Geometry check sheet. Reference: the model listing, model coordinates, mm. A direction names the side the tool comes from. Round coordinates to 2 decimals unless told otherwise and drop trailing zeros. Loops run counter-clockwise (first coordinate to the right, second up) from the corner with the lowest first, then second, coordinate; pieces in that order, holes last. Notation, with made-up numbers: (30.5, 70) - (73.5, 70) arc R26 ccw to (73.5, 105) - close; hole circle Ø6 at (48, -37). An arc over 180 degrees is marked (long way). Answer in a Markdown table with one row per item. Add a question column.
```python
from build123d import *

# Parameters (mm, degrees)
SKETCH4_W           = 17.9705
SKETCH4_H           = 57.023
SKETCH4_W_2         = 1.5875
SKETCH4_H_2         = 16.51
BOSS_EXTRUDE3_DEPTH = 9.906
SKETCH6_W           = 0.762
SKETCH6_H           = 36.957
REVOLVE2_ANGLE      = 345
SKETCH8_W           = 0.635
SKETCH8_H           = 4.826
BOSS_EXTRUDE4_DEPTH = 6.985


with BuildPart() as part:
    # Sketch4 → Revolve1 (revolve)
    with BuildSketch(Plane(origin=(0, 0, 0), x_dir=(0, 0, -1), z_dir=(1, 0, 0))):
        with Locations((8.98525, 28.5115)):
            Rectangle(SKETCH4_W, SKETCH4_H)
        Polygon((0, 61.341), (0, 57.023), (6.477, 57.023), (6.477, 61.341), (1.5875, 61.341), align=None)
        with Locations((0.79375, 69.596)):
            Rectangle(SKETCH4_W_2, SKETCH4_H_2)
    revolve(axis=Axis((0, -9.179219972, 0), (0, 1, 0)))

    # Sketch5 → Boss-Extrude3 (add)
    # profile 1 of 12: a face of its own
    with BuildSketch(Plane(origin=(0, 77.851, 0), x_dir=(1, 0, 0), z_dir=(0, 1, 0))):
        with BuildLine():
            ThreePointArc((-2.91443478, 2.721877799), (-2.343970029, 3.22619797), (-1.688049741, 3.612898686))
            Line((-1.688049741, 3.612898686), (-2.300310076, 4.082888836))
            ThreePointArc((-2.300310076, 4.082888836), (-2.754538028, 3.791296341), (-3.172223127, 3.449406923))
            Line((-3.172223127, 3.449406923), (-2.91443478, 2.721877799))
        make_face()
    # profile 2 of 12: a face of its own
    with BuildSketch(Plane(origin=(0, 77.851, 0), x_dir=(1, 0, 0), z_dir=(0, 1, 0))):
        with BuildLine():
            Line((0, 4.6863), (0, 3.9878))
            ThreePointArc((0, 3.9878), (0.380712775, 3.969585195), (0.757947638, 3.915107178))
            Line((0.757947638, 3.915107178), (0.538871901, 4.655214793))
            ThreePointArc((0.538871901, 4.655214793), (0.269883871, 4.678522244), (0, 4.6863))
        make_face()
    # profile 3 of 12: a face of its own
    with BuildSketch(Plane(origin=(0, 77.851, 0), x_dir=(1, 0, 0), z_dir=(0, 1, 0))):
        with BuildLine():
            Line((-0.538871901, 4.655214793), (-0.757947638, 3.915107178))
            ThreePointArc((-0.757947638, 3.915107178), (-0.380712775, 3.969585195), (0, 3.9878))
            Line((0, 3.9878), (0, 4.6863))
            Line((0, 4.6863), (-0.538871901, 4.655214793))
        make_face()
    # profile 4 of 12: a face of its own
    with BuildSketch(Plane(origin=(0, 77.851, 0), x_dir=(1, 0, 0), z_dir=(0, 1, 0))):
        with BuildLine():
            Line((2.300310076, 4.082888836), (1.688049741, 3.612898686))
            ThreePointArc((1.688049741, 3.612898686), (2.343970029, 3.22619797), (2.91443478, 2.721877799))
            Line((2.91443478, 2.721877799), (3.172223127, 3.449406923))
            ThreePointArc((3.172223127, 3.449406923), (2.754538028, 3.791296341), (2.300310076, 4.082888836))
        make_face()
    # profile 5 of 12: a face of its own
    with BuildSketch(Plane(origin=(0, 77.851, 0), x_dir=(1, 0, 0), z_dir=(0, 1, 0))):
        with BuildLine():
            Line((4.260851788, 1.951038116), (3.489269493, 1.930685693))
            ThreePointArc((3.489269493, 1.930685693), (3.792623176, 1.23229797), (3.957706895, 0.488983613))
            Line((3.957706895, 0.488983613), (4.593892938, 0.926042851))
            ThreePointArc((4.593892938, 0.926042851), (4.456936152, 1.448146341), (4.260851788, 1.951038116))
        make_face()
    # profile 6 of 12: a face of its own
    with BuildSketch(Plane(origin=(0, 77.851, 0), x_dir=(1, 0, 0), z_dir=(0, 1, 0))):
        with BuildLine():
            Line((4.593892938, -0.926042851), (3.957706895, -0.488983613))
            ThreePointArc((3.957706895, -0.488983613), (3.792623176, -1.23229797), (3.489269493, -1.930685693))
            Line((3.489269493, -1.930685693), (4.260851788, -1.951038116))
            ThreePointArc((4.260851788, -1.951038116), (4.456936152, -1.448146341), (4.593892938, -0.926042851))
        make_face()
    # profile 7 of 12: a face of its own
    with BuildSketch(Plane(origin=(0, 77.851, 0), x_dir=(1, 0, 0), z_dir=(0, 1, 0))):
        with BuildLine():
            Line((3.172223127, -3.449406923), (2.91443478, -2.721877799))
            ThreePointArc((2.91443478, -2.721877799), (2.343970029, -3.22619797), (1.688049741, -3.612898686))
            Line((1.688049741, -3.612898686), (2.300310076, -4.082888836))
            ThreePointArc((2.300310076, -4.082888836), (2.754538028, -3.791296341), (3.172223127, -3.449406923))
        make_face()
    # profile 8 of 12: a face of its own
    with BuildSketch(Plane(origin=(0, 77.851, 0), x_dir=(1, 0, 0), z_dir=(0, 1, 0))):
        with BuildLine():
            ThreePointArc((0.757947638, -3.915107178), (0, -3.9878), (-0.757947638, -3.915107178))
            Line((-0.757947638, -3.915107178), (-0.538871901, -4.655214793))
            ThreePointArc((-0.538871901, -4.655214793), (0, -4.6863), (0.538871901, -4.655214793))
            Line((0.538871901, -4.655214793), (0.757947638, -3.915107178))
        make_face()
    # profile 9 of 12: a face of its own
    with BuildSketch(Plane(origin=(0, 77.851, 0), x_dir=(1, 0, 0), z_dir=(0, 1, 0))):
        with BuildLine():
            ThreePointArc((-1.688049741, -3.612898686), (-2.343970029, -3.22619797), (-2.91443478, -2.721877799))
            Line((-2.91443478, -2.721877799), (-3.172223127, -3.449406923))
            ThreePointArc((-3.172223127, -3.449406923), (-2.754538028, -3.791296341), (-2.300310076, -4.082888836))
            Line((-2.300310076, -4.082888836), (-1.688049741, -3.612898686))
        make_face()
    # profile 10 of 12: a face of its own
    with BuildSketch(Plane(origin=(0, 77.851, 0), x_dir=(1, 0, 0), z_dir=(0, 1, 0))):
        with BuildLine():
            ThreePointArc((-3.489269493, -1.930685693), (-3.792623176, -1.23229797), (-3.957706895, -0.488983613))
            Line((-3.957706895, -0.488983613), (-4.593892938, -0.926042851))
            ThreePointArc((-4.593892938, -0.926042851), (-4.456936152, -1.448146341), (-4.260851788, -1.951038116))
            Line((-4.260851788, -1.951038116), (-3.489269493, -1.930685693))
        make_face()
    # profile 11 of 12: a face of its own
    with BuildSketch(Plane(origin=(0, 77.851, 0), x_dir=(1, 0, 0), z_dir=(0, 1, 0))):
        with BuildLine():
            ThreePointArc((-3.957706895, 0.488983613), (-3.792623176, 1.23229797), (-3.489269493, 1.930685693))
            Line((-3.489269493, 1.930685693), (-4.260851788, 1.951038116))
            ThreePointArc((-4.260851788, 1.951038116), (-4.456936152, 1.448146341), (-4.593892938, 0.926042851))
            Line((-4.593892938, 0.926042851), (-3.957706895, 0.488983613))
        make_face()
    # profile 12 of 12: a face of its own
    with BuildSketch(Plane(origin=(0, 77.851, 0), x_dir=(1, 0, 0), z_dir=(0, 1, 0))):
        with BuildLine():
            ThreePointArc((0, 3.9878), (-0.380712775, 3.969585195), (-0.757947638, 3.915107178))
            ThreePointArc((-0.757947638, 3.915107178), (-1.23229797, 3.792623176), (-1.688049741, 3.612898686))
            ThreePointArc((-1.688049741, 3.612898686), (-2.343970029, 3.22619797), (-2.91443478, 2.721877799))
            ThreePointArc((-2.91443478, 2.721877799), (-3.22619797, 2.343970029), (-3.489269493, 1.930685693))
            ThreePointArc((-3.489269493, 1.930685693), (-3.792623176, 1.23229797), (-3.957706895, 0.488983613))
            ThreePointArc((-3.957706895, 0.488983613), (-3.9878, 0), (-3.957706895, -0.488983613))
            ThreePointArc((-3.957706895, -0.488983613), (-3.792623176, -1.23229797), (-3.489269493, -1.930685693))
            ThreePointArc((-3.489269493, -1.930685693), (-3.22619797, -2.343970029), (-2.91443478, -2.721877799))
            ThreePointArc((-2.91443478, -2.721877799), (-2.343970029, -3.22619797), (-1.688049741, -3.612898686))
            ThreePointArc((-1.688049741, -3.612898686), (-1.23229797, -3.792623176), (-0.757947638, -3.915107178))
            ThreePointArc((-0.757947638, -3.915107178), (0, -3.9878), (0.757947638, -3.915107178))
            ThreePointArc((0.757947638, -3.915107178), (1.23229797, -3.792623176), (1.688049741, -3.612898686))
            ThreePointArc((1.688049741, -3.612898686), (2.343970029, -3.22619797), (2.91443478, -2.721877799))
            ThreePointArc((2.91443478, -2.721877799), (3.22619797, -2.343970029), (3.489269493, -1.930685693))
            ThreePointArc((3.489269493, -1.930685693), (3.792623176, -1.23229797), (3.957706895, -0.488983613))
            ThreePointArc((3.957706895, -0.488983613), (3.980269614, -0.244954368), (3.9878, 0))
            ThreePointArc((3.9878, 0), (3.980269614, 0.244954368), (3.957706895, 0.488983613))
            ThreePointArc((3.957706895, 0.488983613), (3.792623176, 1.23229797), (3.489269493, 1.930685693))
            ThreePointArc((3.489269493, 1.930685693), (3.22619797, 2.343970029), (2.91443478, 2.721877799))
            ThreePointArc((2.91443478, 2.721877799), (2.343970029, 3.22619797), (1.688049741, 3.612898686))
            ThreePointArc((1.688049741, 3.612898686), (1.23229797, 3.792623176), (0.757947638, 3.915107178))
            ThreePointArc((0.757947638, 3.915107178), (0.380712775, 3.969585195), (0, 3.9878))
        make_face()
        with BuildLine():
            ThreePointArc((0, -1.5875), (-1.5875, 0), (0, 1.5875))
            ThreePointArc((0, 1.5875), (1.122532015, 1.122532015), (1.5875, 0))
            ThreePointArc((1.5875, 0), (1.122532015, -1.122532015), (0, -1.5875))
        make_face(mode=Mode.SUBTRACT)
    extrude(amount=-BOSS_EXTRUDE3_DEPTH)

    # Sketch6 → Revolve2 (revolve)
    with BuildSketch(Plane(origin=(0, 0, 0), x_dir=(0, 0, -1), z_dir=(1, 0, 0))):
        with Locations((18.3515, 36.0045)):
            Rectangle(SKETCH6_W, SKETCH6_H)
    revolve(axis=Axis((0, 0, 0), (0, 1, 0)), revolution_arc=REVOLVE2_ANGLE)

    # Sketch8 → Boss-Extrude4 (add)
    with BuildSketch(Plane.XZ):
        with Locations((-13.97, 0.523045405)):
            Rectangle(SKETCH8_W, SKETCH8_H)
        with Locations((13.97, 0.523045405)):
            Rectangle(SKETCH8_W, SKETCH8_H)
    extrude(amount=BOSS_EXTRUDE4_DEPTH)


solid = part.part
```
Q1. Cross-section at C-C, the plane x = 16. Enter the section's corners in (y, z), plus the area to 3 significant figures.
Q2. Set-up check for faces 1 (the flat face through (-13.652, -3, 0)), 2 (the flat face through (0, 57.023, 8)), 3 (the flat face through (2, 67.945, 0)), 4 (the flat face through (-14.288, -3, 0)): record each of +Z, -Z, +X, -X, +Y, -Y from which the full face is reachable in a straight line by a thin tool's end or side.
Q3. Scan lines: line 1 (Y direction, x = -2.5, z = 3) (3 decimals); line 2 (Y direction, x = -11.5, z = -3.5); line 3 (Y direction, x = -2, z = 6). Record each from-to range of solid material in increasing order. Write a range as from..to.
Q4. Depth check by flat-ended pin: P1, Ø1, axis at x = -6, z = 14.5, coming from the +Y side; P2, Ø8, axis at x = 2, z = -6.5, coming from the -Y side; P3, Ø0.7, axis at x = 14, y = -2, coming from the -Z side. Enter the tip coordinate at first touch or a pass-through.
Q5. Cross-section at B-B, the plane y = 45.5. Enter the section's corners in (x, z) (1 decimal).
Q6. Release check for a two-part mould opening along X. For faces 5 (the flat face through (13.652, -3, 0)), 6 (the flat face through (-7, 54.483, 17)), 7 (the flat face through (14.288, -3, 0)) record: +X half, -X half, draft (parallel to the pull), parting line (faces both ways), or undercut.
Q7. Cross-section at D-D, the plane y = 1.5. Enter the section's corners in (x, z).
Q8. Cross-section at A-A, the plane z = -15.5. Enter the section's corners in (x, y).
Check sheet entries:
| question | item | result |
|---|---|---|
| 1 | outline | (0, -8.18) - (17.53, -8.18) - (17.53, -9.74) - (54.48, -9.74) - (54.48, -8.18) - (57.02, -8.18) - (57.02, 8.18) - (54.48, 8.18) - (54.48, 9.74) - (17.53, 9.74) - (17.53, 8.18) - (0, 8.18) - close |
| 1 | area | 1,050 mm² |
| 2 | face 1 | +Z, -Z, -Y |
| 2 | face 2 | +Y |
| 2 | face 3 | none |
| 2 | face 4 | +Z, -Z, -X, -Y |
| 3 | line 1 | 0..61.341, 67.945..77.851 |
| 3 | line 2 | 0..57.02 |
| 3 | line 3 | 0..61.34 |
| 4 | P1 | y = 57.02 |
| 4 | P2 | y = 0 |
| 4 | P3 | z = -1.89 |
| 5 | outline | (0, -18.7) - (0, -18) arc R18 ccw to (4.7, -17.4) - (4.8, -18.1) arc R18.7 ccw (long way) to start |
| 6 | face 5 | undercut |
| 6 | face 6 | draft |
| 6 | face 7 | +X half |
| 7 | outline | circle Ø35.94 at (0, 0) |
| 8 | outline | (-10.52, 17.53) - (-9.09, 17.53) - (-9.09, 0) - (9.09, 0) - (9.09, 17.53) - (10.52, 17.53) - (10.52, 54.48) - (9.09, 54.48) - (9.09, 57.02) - (-9.09, 57.02) - (-9.09, 54.48) - (-10.52, 54.48) - close |
